Job drawing, mm, ordinate dimensions from the low corner. One solid piece. A direction names the side the tool comes from. Round coordinates to 2 decimals unless told otherwise and drop trailing zeros. Loops run counter-clockwise (first coordinate to the right, second up) from the corner with the lowest first, then second, coordinate; pieces in that order, holes last. Notation, with made-up numbers: M 2.25,64 L 7.25,64 A17 cw 7.25,72 Z; hole C 20.5,-35 d9. An arc over 180 degrees is marked long. Use a Markdown table: item, result. Add a question column.
(1) Wall check: L1, parallel to Z at x = 6.5, y = 23; L2, parallel to X at y = 20, z = 11; L3, parallel to Y at x = 21.75, z = 15.75. Give the ranges that are in metal, low to high.
(2) Which spindle directions (+Z, -Z, +X, -X, +Y, -Y) get a long thin tool onto all of the face, cutting with end or side? Do the marked faces 1, 2 and 3. Say none if no direction does.
(3) Band-saw the part on C-C, the plane x = 7.5. Write the cut outline in (y, z), and give its area (4 significant figures).
(4) Flat gauge pins, fed straight in: P1, Ø12, axis at x = 8.5, y = 18.5, coming from the +Z side; P2, Ø1.5, axis at x = 13.5, z = 8, coming from the -Y side (3 decimals); P3, Ø10, axis at x = 7.5, z = 3.5, coming from the -Y side. Where does each tip first touch, or does it go through?
(5) Band-saw the part on B-B, the plane z = 7.25. Write the cut outline in (x, y).
(6) Band-saw the part on A-A, the plane y = 18.5. Write the cut outline in (x, z).
(7) Band-saw the part on D-D, the plane z = 13. Write the cut outline in (x, y), and give its area (3 significant figures).
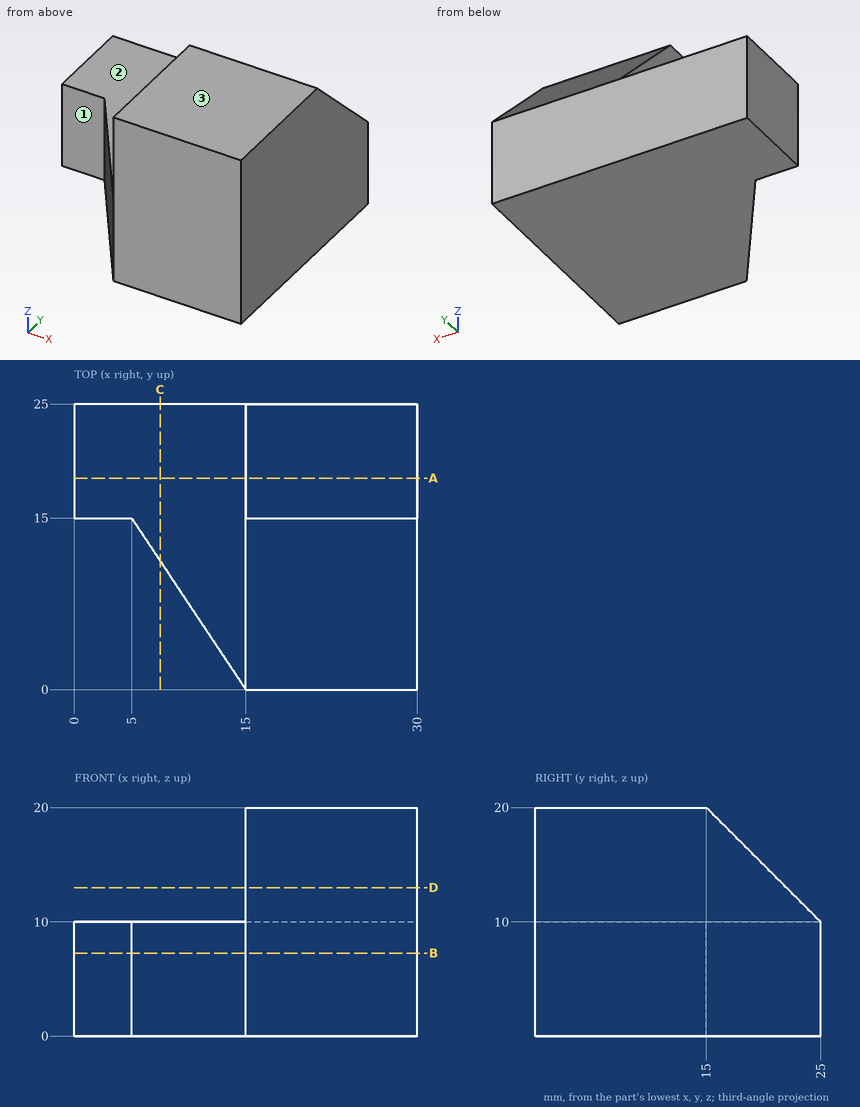
Return value:
| question | item | result |
|---|---|---|
| 1 | L1 | 0 to 10 |
| 1 | L2 | 15 to 30 |
| 1 | L3 | 0 to 19.25 |
| 2 | face 1 | +Z, -Z, -X, -Y |
| 2 | face 2 | +Z, -X, +Y, -Y |
| 2 | face 3 | +Z, +X, -X, +Y, -Y |
| 3 | outline | M 11.25,0 L 25,0 L 25,10 L 11.25,10 Z |
| 3 | area | 137.5 mm^2 |
| 4 | P1 | z = 10 |
| 4 | P2 | y = 1.125 |
| 4 | P3 | y = 3.75 |
| 5 | outline | M 0,15 L 5,15 L 15,0 L 30,0 L 30,25 L 0,25 Z |
| 6 | outline | M 0,0 L 30,0 L 30,16.5 L 15,16.5 L 15,10 L 0,10 Z |
| 7 | outline | M 15,0 L 30,0 L 30,22 L 15,22 Z |
| 7 | area | 330 mm^2 |
